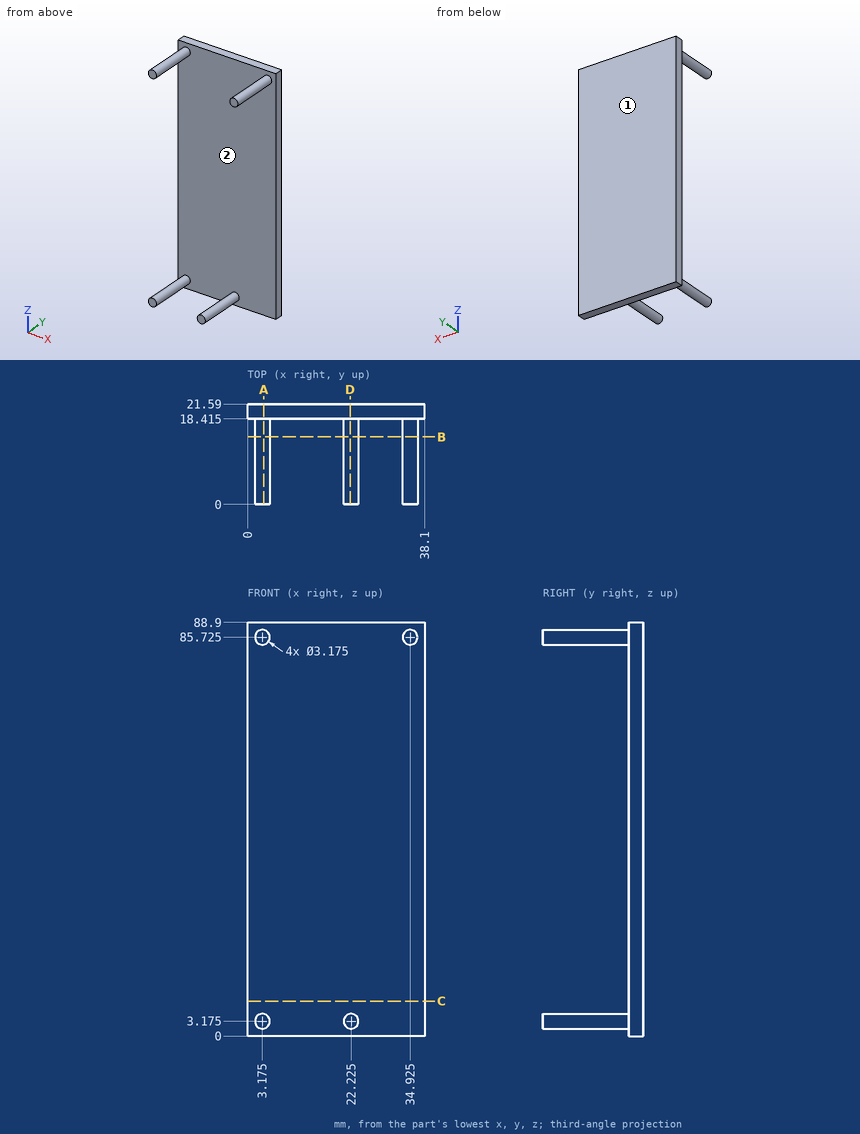
Geometry check sheet. Reference: drawing and pictorial views, mm from the part's lowest x, y, z. Round coordinates to 2 decimals unless told otherwise and drop trailing zeros. Order: outer loops, then holes, each group sorted by start corner. A loop starts at its lowest first (then second) coordinate and runs counter-clockwise, first axis right, second up. Notation, with made-up numbers: M 85.25,-27 L 123.25,-27 A19 cw 123.25,-5 Z; hole C -38,12.5 d2. An arc over 180 degrees is marked long. Answer in a Markdown table with one row per item.
(1) Go/stop test with flat-tipped pins: P1, Ø6, axis at x = 16, z = 57.5, coming from the -Y side (3 decimals); P2, Ø2, axis at x = 22, y = 11, coming from the +Z side; P3, Ø8, axis at y = 11.5, z = 21.5, coming from the +X side. Record where each tip stops, or that it passes through.
Responses:
| item | result |
|---|---|
| P1 | stops at y = 18.415 |
| P2 | stops at z = 4.76 |
| P3 | passes through |
(2) Sectioned sample at A-A, the plane x = 3.5. Record the cut outline in (y, z) (3 decimals), and give its area (3 significant figures).
Responses:
| item | result |
|---|---|
| outline | M 0,1.621 L 18.415,1.621 L 18.415,0 L 21.59,0 L 21.59,88.9 L 18.415,88.9 L 18.415,87.279 L 0,87.279 L 0,84.171 L 18.415,84.171 L 18.415,4.729 L 0,4.729 Z |
| area | 397 mm² |
(3) Draft check along Y on the marked faces 1 and 2. Enter one of: released by +Y, released by -Y, zero draft, split by the parting line, or undercut.
Responses:
| item | result |
|---|---|
| face 1 | released by +Y |
| face 2 | released by -Y |
(4) Scan lines: probe 1 along Y at (x, z) = (19.5, 79.5) (3 decimals); probe 2 along Z at (x, y) = (22, 1.25). Record each from-to range of solid material in increasing order. Write a range as from..to.
Responses:
| item | result |
|---|---|
| probe 1 | y = 18.415..21.59 |
| probe 2 | z = 1.6..4.75 |
(5) Sectioned sample at D-D, the plane x = 22. Record the cut outline in (y, z) (3 decimals).
Responses:
| item | result |
|---|---|
| outline | M 0,1.604 L 18.415,1.604 L 18.415,0 L 21.59,0 L 21.59,88.9 L 18.415,88.9 L 18.415,4.746 L 0,4.746 Z |
(6) Sectioned sample at B-B, the plane y = 14.5. Record the cut outline in (x, z) (1 decimal), and give its area (3 significant figures).
Responses:
| item | result |
|---|---|
| outline | C 3.2,3.2 d3.2; C 3.2,85.7 d3.2; C 22.2,3.2 d3.2; C 34.9,85.7 d3.2 |
| area | 31.7 mm² |
(7) Sectioned sample at C-C, the plane z = 7.5. Record the cut outline in (x, y) (3 decimals), and give its area (3 significant figures).
Responses:
| item | result |
|---|---|
| outline | M 0,18.415 L 38.1,18.415 L 38.1,21.59 L 0,21.59 Z |
| area | 121 mm² |
